CAD build for the part. Positions are in the model's coordinates, mm. A direction names the side the tool comes from. Round coordinates to 2 decimals unless told otherwise and drop trailing zeros. Order: outer loops, then holes, each group sorted by start corner. A loop starts at its lowest first (then second) coordinate and runs counter-clockwise, first axis right, second up. Notation, with made-up numbers: (13.5, 24) -> (55.5, 24) arc R13 cw to (55.5, 47) -> close; hole circle Ø2 at (77.25, -23.75). An arc over 180 degrees is marked (long way). Return JSON: item names as keys, results as strings. Group by question number.
Q1. Cut at A-A (z = 375.5). Write the cut outline in (x, y).
Q2. Flat gauge pin, fed straight in: pin 1 (3.5 mm diameter, centred on y = 0, z = 670, fed in from +X). Where does the tip first touch, or does it go through?
Q3. Mould opens along X. For faces 1 (the flat face through (-8, 0, 478)), 2 (the flat face through (0, 10, 478)), 3 (the flat face through (0, -8, 478)), 4 (the flat face through (10, 0, 478)) say: +X half, -X half, draft (parallel to the pull), parting line (faces both ways), or undercut.
Q4. Which spindle directions (+Z, -Z, +X, -X, +Y, -Y) get a long thin tool onto all of the face, cutting with end or side? Do faces 5 (the flat face through (-9, 0, 970)), 6 (the flat face through (0, 8, 478)). Say none if no direction does.
Q5. Probe line 1 along X through (y, z) = (-7, 370); line 2 along Z through (x, y) = (-1, 8.75). List the from-to ranges inside material, lowest first.
from build123d import *

# Parameters (mm, degrees)
SKETCH_1_W          = 20
SKETCH_1_H          = 20
SKETCH_1_W_2        = 16
SKETCH_1_H_2        = 16
EXTRUDE_1_DEPTH     = 970
SKETCH_2_R          = 2.2
SKETCH_2_R_2        = 5.5
CUT_EXTRUDE_1_DEPTH = 970
SKETCH_3_R          = 2.2
CUT_EXTRUDE_2_DEPTH = 970
SKETCH_5_R          = 2.2
CUT_EXTRUDE_4_DEPTH = 30


with BuildPart() as part:
    # ｽｹｯﾁ1 → ﾎﾞｽ - 押し出し1 (new body)
    with BuildSketch(Plane.XY):
        Rectangle(SKETCH_1_W, SKETCH_1_H)
        Rectangle(SKETCH_1_W_2, SKETCH_1_H_2, mode=Mode.SUBTRACT)
    extrude(amount=EXTRUDE_1_DEPTH)

    # ｽｹｯﾁ2 → ｶｯﾄ - 押し出し1 (cut)
    with BuildSketch(Plane(origin=(10, 0, 0), x_dir=(0, 0, -1), z_dir=(1, 0, 0))):
        with Locations((-710, 0)):
            Circle(SKETCH_2_R)
        with Locations((-670, 0)):
            Circle(SKETCH_2_R)
        with Locations((-50, 0)):
            Circle(SKETCH_2_R_2)
        with Locations((-30, 0)):
            Circle(SKETCH_2_R)
    extrude(amount=-CUT_EXTRUDE_1_DEPTH, mode=Mode.SUBTRACT)

    # ｽｹｯﾁ3 → ｶｯﾄ - 押し出し2 (cut)
    with BuildSketch(Plane(origin=(0, 10, 0), x_dir=(1, 0, 0), z_dir=(0, 1, 0))):
        with Locations((0, -690)):
            Circle(SKETCH_3_R)
        with Locations((0, -660)):
            Circle(SKETCH_3_R)
        with Locations((0, -10)):
            Circle(SKETCH_3_R)
    extrude(amount=-CUT_EXTRUDE_2_DEPTH, mode=Mode.SUBTRACT)

    # ｽｹｯﾁ5 → ｶｯﾄ - 押し出し4 (cut)
    with BuildSketch(Plane(origin=(0, 10, 0), x_dir=(1, 0, 0), z_dir=(0, 1, 0))):
        with Locations((0, -110)):
            Circle(SKETCH_5_R)
        with Locations((0, -139)):
            Circle(SKETCH_5_R)
    extrude(amount=-CUT_EXTRUDE_4_DEPTH, mode=Mode.SUBTRACT)


solid = part.part
Solution:
{
 "1": {"outline": "(-10, -10) -> (10, -10) -> (10, 10) -> (-10, 10) -> close; hole (-8, -8) -> (8, -8) -> (8, 8) -> (-8, 8) -> close"},
 "2": {"pin 1": "passes through"},
 "3": {"face 1": "undercut", "face 2": "draft", "face 3": "undercut", "face 4": "+X half"},
 "4": {"face 5": "+Z, +X, -X, +Y, -Y", "face 6": "+Z, -Z"},
 "5": {"line 1": "x = -10 to -8, 8 to 10", "line 2": "z = 0 to 8.04, 11.96 to 108.04, 111.96 to 137.04, 140.96 to 658.04, 661.96 to 688.04, 691.96 to 970"}
}
